```python
from build123d import *

# Parameters (mm, degrees)
ESBO_O2_R                = 3
RESSALTO_EXTRUS_O1_DEPTH = 5
ESBO_O11_R               = 5
CORTE_EXTRUS_O3_DEPTH    = 2
ESBO_O3_W                = 45
ESBO_O3_H                = 13
RESSALTO_EXTRUS_O2_DEPTH = 10
ESBO_O4_W                = 45
ESBO_O4_H                = 20
RESSALTO_EXTRUS_O3_DEPTH = 17
ESBO_O6_W                = 30.5
ESBO_O6_H                = 6.5
CORTE_EXTRUS_O1_DEPTH    = 15
ESBO_O7_W                = 45
ESBO_O7_H                = 5
RESSALTO_EXTRUS_O4_DEPTH = 50
ESBO_O8_W                = 45
ESBO_O8_H                = 15
RESSALTO_EXTRUS_O5_DEPTH = 15
ESBO_O9_W                = 35.5
ESBO_O9_H                = 5.5
CORTE_EXTRUS_O2_DEPTH    = 15
FILETE4_R                = 5
FILETE6_R                = 15
FILETE7_R                = 2


with BuildPart() as part:
    # Esboço2 → Ressalto-extrusão1 (new body)
    with BuildSketch(Plane.XY):
        with BuildLine():
            Line((-22.5, 0), (-22.5, 30))
            Line((-22.5, 30), (22.5, 30))
            Line((22.5, 30), (22.5, 0))
            ThreePointArc((22.5, 0), (0, -22.5), (-22.5, 0))
        make_face()
        Circle(ESBO_O2_R, mode=Mode.SUBTRACT)
    extrude(amount=RESSALTO_EXTRUS_O1_DEPTH)

    # Esboço11 → Corte-extrusão3 (cut)
    with BuildSketch(Plane.XY.offset(5)):
        Circle(ESBO_O11_R)
    extrude(amount=-CORTE_EXTRUS_O3_DEPTH, mode=Mode.SUBTRACT)

    # Esboço3 → Ressalto-extrusão2 (add)
    with BuildSketch(Plane(origin=(0, 0, 0), x_dir=(-1, 0, 0), z_dir=(0, 0, -1))):
        with Locations((0, 23.5)):
            Rectangle(ESBO_O3_W, ESBO_O3_H)
    extrude(amount=RESSALTO_EXTRUS_O2_DEPTH)

    # Esboço4 → Ressalto-extrusão3 (add)
    with BuildSketch(Plane(origin=(0, 30, 0), x_dir=(1, 0, 0), z_dir=(0, 1, 0))):
        with Locations((0, 5)):
            Rectangle(ESBO_O4_W, ESBO_O4_H)
    extrude(amount=RESSALTO_EXTRUS_O3_DEPTH)

    # Esboço6 → Corte-extrusão1 (cut)
    with BuildSketch(Plane(origin=(0, 0, -15), x_dir=(-1, 0, 0), z_dir=(0, 0, -1))):
        with Locations((0, 38.5)):
            Rectangle(ESBO_O6_W, ESBO_O6_H)
    extrude(amount=-CORTE_EXTRUS_O1_DEPTH, mode=Mode.SUBTRACT)

    # Esboço7 → Ressalto-extrusão4 (add)
    with BuildSketch(Plane(origin=(0, 47, 0), x_dir=(1, 0, 0), z_dir=(0, 1, 0))):
        with Locations((0, -2.5)):
            Rectangle(ESBO_O7_W, ESBO_O7_H)
    extrude(amount=RESSALTO_EXTRUS_O4_DEPTH)

    # Esboço8 → Ressalto-extrusão5 (add)
    with BuildSketch(Plane(origin=(0, 0, 0), x_dir=(-1, 0, 0), z_dir=(0, 0, -1))):
        with Locations((0, 89.5)):
            Rectangle(ESBO_O8_W, ESBO_O8_H)
    extrude(amount=RESSALTO_EXTRUS_O5_DEPTH)

    # Esboço9 → Corte-extrusão2 (cut)
    with BuildSketch(Plane(origin=(0, 0, -15), x_dir=(-1, 0, 0), z_dir=(0, 0, -1))):
        with Locations((0, 89.5)):
            Rectangle(ESBO_O9_W, ESBO_O9_H)
    extrude(amount=-CORTE_EXTRUS_O2_DEPTH, mode=Mode.SUBTRACT)

    # Filete4
    filete4_edges = [part.edges().sort_by_distance(p)[0] for p in [
        (0, 30, -10),
    ]]
    fillet(filete4_edges, radius=FILETE4_R - 0.0001)  # a hair under: the kernel refuses the full size

    # Filete6
    filete6_edges = [part.edges().sort_by_distance(p)[0] for p in [
        (0, 82, 0),
    ]]
    fillet(filete6_edges, radius=FILETE6_R - 0.0001)  # a hair under: the kernel refuses the full size

    # Filete7
    filete7_edges = [part.edges().sort_by_distance(p)[0] for p in [
        (-5, 0, 5),
    ]]
    fillet(filete7_edges, radius=FILETE7_R - 0.0001)  # a hair under: the kernel refuses the full size


solid = part.part
```
Can you work these out from the model? Positions are in its coordinate system, mm. A direction names the side the tool comes from. Coordinates: 2 decimals unless noted, no trailing zeros. Loops run counter-clockwise (first coordinate to the right, second up) from the corner with the lowest first, then second, coordinate; pieces in that order, holes last. Notation, with made-up numbers: M -4.5,38.25 L 34.5,38.25 A13 ccw 34.5,62.25 Z; hole C -25,13 d4. An arc over 180 degrees is marked long. Put each result on its own line as item: value. Start each with the question number.
(1) Will these pins go through, and if not, where does the flat tip stop? pin 1 Ø8 at (x, y) = (0, 2) entering from +Z; pin 2 Ø8 at (x, y) = (-11, 0) entering from -Z; pin 3 Ø2 at (x, z) = (-17, -12) entering from -Y; pin 4 Ø3.5 at (x, y) = (0, 0) entering from +Z.
(2) Imagine slicing it at C-C on y = 40. List the corners of the cut face in (x, z) for me, and give its area (4 significant figures).
(3) Which directions (+Z, -Z, +X, -X, +Y, -Y) give clear straight access to the entire face, cutting with the end or side of a thin tool? Please do faces 1 (the face through (0, 21, -10)), 2 (the face through (0, 86.75, -8)), 3 (the face through (-0.1, -3.3, 3)).
(4) Imagine slicing it at A-A on z = -2.5. List the corners of the cut face in (x, y) for me, and give its area (3 significant figures).
(5) We'd pull the mould along Y, two halves only. Please class faces 4 (the face through (0, 47, -8)), 5 (the face through (0, 17, -5)), 6 (the face through (0, 86, -15)): +Y half, -Y half, draft (parallel to the pull), parting line (faces both ways), or undercut.
(6) I need wall thicknesses on probe 1 along X at (y, z) = (0, 1.3); probe 2 along Y at (x, z) = (0, 2.1); probe 3 along Y at (x, z) = (3, -13.25). Which ranges of each line are inside material? Lowest first, please.
Worked answers:
1. pin 1: stops at z = 4.73
1. pin 2: stops at z = 0
1. pin 3: stops at y = 28
1. pin 4: passes through
2. outline: M -22.5,-15 L -15.25,-15 L -15.25,0 L 15.25,0 L 15.25,-15 L 22.5,-15 L 22.5,5 L -22.5,5 Z
2. area: 442.5 mm2
3. face 1: -Z, +X, -X, -Y
3. face 2: -Z
3. face 3: +Z
4. outline: M -22.5,17 L 22.5,17 L 22.5,47 L -22.5,47 Z; M -22.5,75.29 L 22.5,75.29 L 22.5,97 L -22.5,97 Z; hole M -17.75,86.75 L 17.75,86.75 L 17.75,92.25 L -17.75,92.25 Z; hole M -15.25,35.25 L 15.25,35.25 L 15.25,41.75 L -15.25,41.75 Z
4. area: 1,930 mm2
5. face 4: undercut
5. face 5: -Y half
5. face 6: draft
6. probe 1: x = -22.5 to -3, 3 to 22.5
6. probe 2: y = -22.5 to -3, 3 to 97
6. probe 3: y = 29.68 to 35.25, 41.75 to 47, 81.9 to 86.75, 92.25 to 97
